Autodesk Inventor part; units mm, degrees
ref_plane "YZ Plane" through (0, 0, 0) normal (1, 0, 0) x (0, 1, 0)
ref_plane "XZ Plane" through (0, 0, 0) normal (0, 1, 0) x (-1, 0, 0)
ref_plane "XY Plane" through (0, 0, 0) normal (0, 0, 1) x (1, 0, 0)
sketch "スケッチ1" plane through (0, 0, 0) normal (0, 0, 1) x (1, 0, 0)
  line L0 (5, 2.8868) -> (22.5, 12.9904)
  line L1 (22.5, 12.9904) -> (-22.5, 12.9904)
  line L2 (-22.5, 12.9904) -> (-5, 2.8868)
  line L3 (-22.5, 12.9904) -> (-22.5, 14.9904)
  line L4 (-22.5, 14.9904) -> (-25, 14.9904)
  line L5 (-25, 14.9904) -> (-25, 12.9904)
  line L6 (-25, 12.9904) -> (-26.5, 12.9904)
  line L7 (-26.5, 12.9904) -> (-26.5, 16.9904)
  line L8 (-26.5, 16.9904) -> (26.5, 16.9904)
  line L9 (26.5, 16.9904) -> (26.5, 12.9904)
  line L10 (26.5, 12.9904) -> (25, 12.9904)
  line L11 (25, 12.9904) -> (25, 14.9904)
  line L12 (25, 14.9904) -> (22.5, 14.9904)
  line L13 (22.5, 14.9904) -> (22.5, 12.9904)
  line L14 (-22.5, 14.9904) -> (-22.5, 54.9904)
  line L15 (-22.5, 54.9904) -> (22.5, 54.9904)
  line L16 (22.5, 54.9904) -> (22.5, 14.9904)
  arc A0 (-5, 2.8868) -> (5, 2.8868) centre (0, 11.547) ccw
  line L17 (0, 0) -> (0, 54.9904)
  line L18 (-25, 12.9904) -> (-25, 4.9904)
  line L19 (-25, 4.9904) -> (-26.5, 4.9904)
  line L20 (-26.5, 4.9904) -> (-26.5, 12.9904)
  line L21 (25, 12.9904) -> (25, 4.9904)
  line L22 (25, 4.9904) -> (26.5, 4.9904)
  line L23 (26.5, 4.9904) -> (26.5, 12.9904)
  point P0 (0, 1.547)
  point P1 (0, 16.9904)
  dimension "d0" = 45
  dimension "d1" = 30
  dimension "d2" = 2.5
  dimension "d3" = 1.5
  dimension "d4" = 2
  dimension "d5" = 4
  dimension "d6" = 40
  dimension "d7" = 10
  dimension "d9" = 8
  dimension "d10" = 50
revolve "回転1" add sketch "スケッチ1" angle 360 about axis through (0, 0, 0) along (0, 1, 0) contours A0 L17 L1 L0 | L1 L17 L8 L16 L13 | L16 L8 L9 L10 L11 L12
fillet "フィレット1" radius 1 2 edges at (-25, 12.9904, 0) (-22.5, 12.9904, 0)
properties part number "COne_mirror"
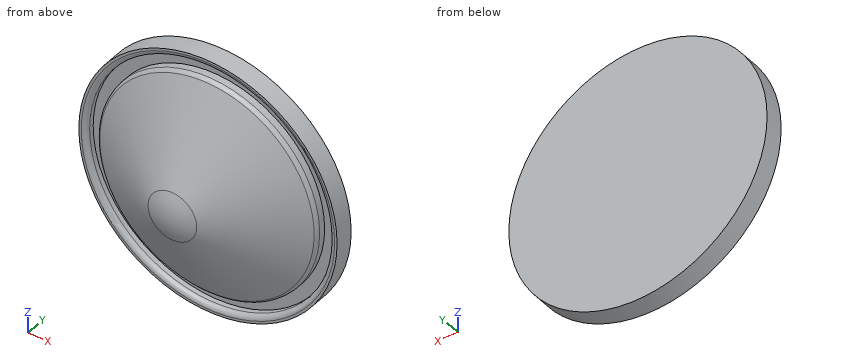
The listing builds one solid part. Answer for the finished solid, in the listing's coordinates (mm). Coordinates: 2 decimals unless noted, no trailing zeros. Loops run counter-clockwise (first coordinate to the right, second up) from the corner with the lowest first, then second, coordinate; pieces in that order, holes last. Notation, with made-up numbers: M 51,70.25 L 78,70.25 A19 ccw 78,84.25 Z; hole C 50,-1.5 d3. An arc over 180 degrees is marked long. Answer as a JSON object with one key per item and string values. Group by question number.
Item 1: Consider L1, parallel to X at y = 14.6, z = 0; L2, parallel to Y at x = 18, z = -16.5. Determine where each line is inside the solid, lowest interval first.
Item 2: Section A-A (y = 5.75) is taken. Write down the section's boundary in (x, z).
Item 3: Each of these flat-tipped pins is pushed along its axis until it touches: P1, Ø1.5, axis at x = 14.5, z = -20, coming from the -Y side; P2, Ø15, axis at x = 5.5, z = -6, coming from the -Y side; P3, Ø2, axis at y = 13.5, z = -17.5, coming from the -X side. Where does it stop, or does it pass through?
Item 4: Section B-B (y = 10.5) is taken. Write down the section's boundary in (x, z).
Solved:
{
 "1": {"L1": "x = -26.5 to -25, -22.5 to 22.5, 25 to 26.5", "L2": "y = 14.99 to 16.99"},
 "2": {"outline": "C 0,0 d19.92"},
 "3": {"P1": "stops at y = 13.15", "P2": "stops at y = 1.57", "P3": "stops at x = -20.74"},
 "4": {"outline": "C 0,0 d36.37"}
}
